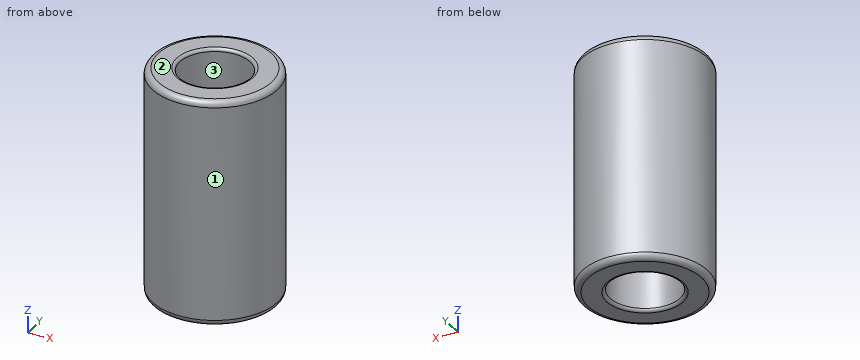
from build123d import *

# Parameters (mm, degrees)
F0_R     = 26.67
F1_DEPTH = 96.52
F2_R     = 14.986
F3_DEPTH = 96.521
F4_R     = 2.54
F5_R     = 1.27


with BuildPart() as f1:
    # F0 (on Top) → F1 (new body)
    with BuildSketch(Plane.XY):
        Circle(F0_R)
    extrude(amount=F1_DEPTH)

    # F2 (on face) → F3 (cut, through all)
    with BuildSketch(Plane.XY.offset(96.52)):
        Circle(F2_R)
    extrude(amount=-F3_DEPTH, mode=Mode.SUBTRACT)

    # F4
    f4_edges = [f1.edges().sort_by_distance(p)[0] for p in [
        (-26.67, 0, 0),
        (-26.67, 0, 96.52),
    ]]
    fillet(f4_edges, radius=F4_R)

    # F5
    f5_edges = [f1.edges().sort_by_distance(p)[0] for p in [
        (-14.986, 0, 96.52),
        (-14.986, 0, 0),
    ]]
    fillet(f5_edges, radius=F5_R)


solid = f1.part
Geometry: final body of the model. Coordinates: model frame, mm. Face numbers are marked on the shaded views. Round coordinates to 2 decimals unless told otherwise and drop trailing zeros. Loops run counter-clockwise (first coordinate to the right, second up) from the corner with the lowest first, then second, coordinate; pieces in that order, holes last. Notation, with made-up numbers: (30.25, 38) - (85.25, 38) arc R13 ccw to (85.25, 45) - close; hole circle Ø5 at (56, 9). An arc over 180 degrees is marked (long way). Write each question's results on one line, items separated by ' | '. Start each with the question number.
1) Line query: probe 1 along Y at (x, z) = (0, 60); probe 2 along Y at (x, z) = (-10, 88); probe 3 along X at (y, z) = (-1, 12). Output: solid intervals per line, ascending. Write a range as [from, to].
2) First-contact query: P1, Ø1.5, axis at x = 5.5, y = 15.5, coming from the -Z side; P2, Ø10, axis at x = 20.5, z = 26.5, coming from the -Y side; P3, Ø3, axis at x = 0, z = 47.5, coming from the +Y side; P4, Ø8, axis at x = 3, z = 52, coming from the -Y side. Flat tips, straight axial feed; report the tip coordinate or a pass-through.
3) Cut plane C-C on z = 25.5. Return loops of the section in (x, y).
4) Cut plane A-A on y = 0. Return loops of the section in (x, z).
5) Mould query, pull axis Y, two halves, no side actions, for the marked faces 1, 2 and 3. Classes: released by +Y, released by -Y, zero draft, split by the parting line, or undercut.
Verdict:
1) probe 1: y = [-26.67, -14.99], [14.99, 26.67] | probe 2: y = [-24.72, -11.16], [11.16, 24.72] | probe 3: x = [-26.65, -14.95], [14.95, 26.65]
2) P1: stops at z = 0 | P2: stops at y = -21.7 | P3: stops at y = 26.67 | P4: stops at y = -26.67
3) outline: circle Ø53.34 at (0, 0); hole circle Ø29.97 at (0, 0)
4) outline: (-26.67, 2.54) arc R2.54 ccw to (-24.13, 0) - (-16.26, 0) arc R1.27 ccw to (-14.99, 1.27) - (-14.99, 95.25) arc R1.27 ccw to (-16.26, 96.52) - (-24.13, 96.52) arc R2.54 ccw to (-26.67, 93.98) - close; (14.99, 1.27) arc R1.27 ccw to (16.26, 0) - (24.13, 0) arc R2.54 ccw to (26.67, 2.54) - (26.67, 93.98) arc R2.54 ccw to (24.13, 96.52) - (16.26, 96.52) arc R1.27 ccw to (14.99, 95.25) - close
5) face 1: split by the parting line | face 2: zero draft | face 3: undercut
